For this review, use the dimensioned drawing (mm, ordinates from the lowest corner) and the shaded views. Give positions to 0.01 mm unless a question says otherwise; leave off trailing zeros. Order: outer loops, then holes, each group sorted by start corner. A loop starts at its lowest first (then second) coordinate and runs counter-clockwise, first axis right, second up. Notation, with made-up numbers: (10, 64) -> (68, 64) arc R19 ccw to (68, 98) -> close; hole circle Ø11 at (-32.5, -9). An arc over 180 degrees is marked (long way). Return JSON: item names as keys, results as strings.
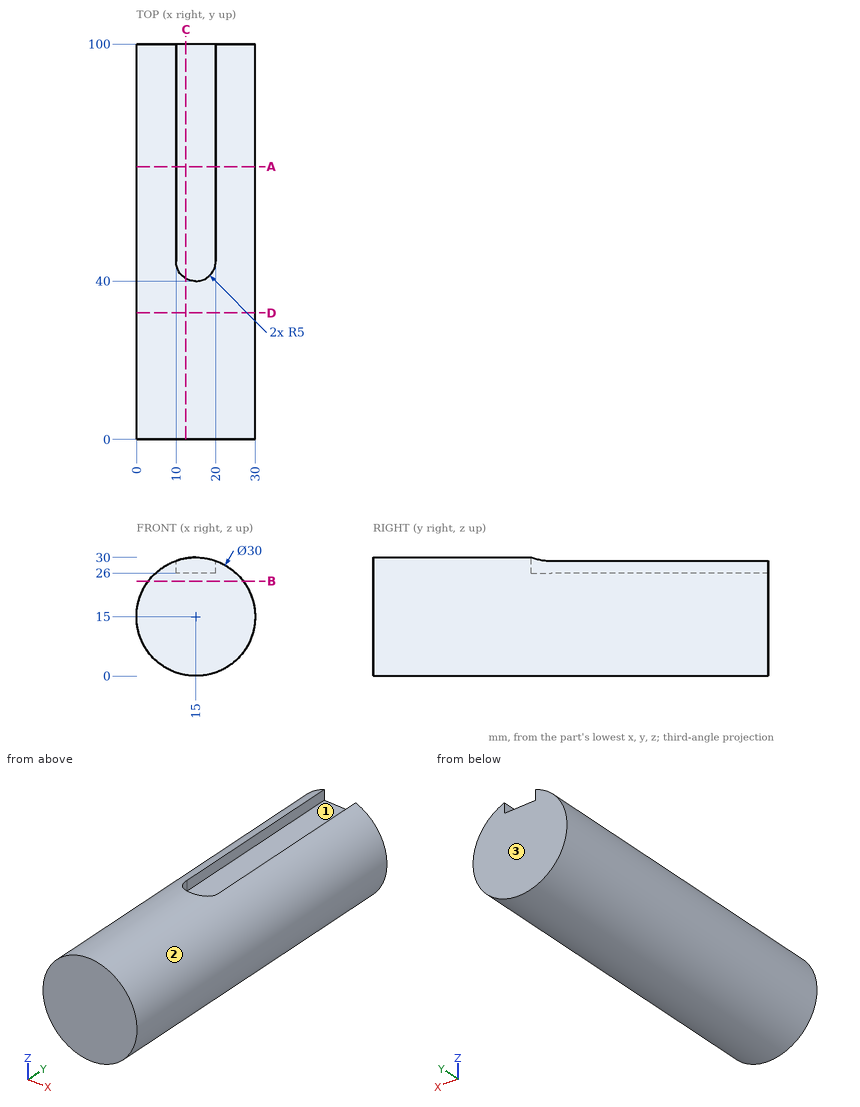
Item 1: Mouldability with a two-part tool opening along X and no side actions: class the marked faces 1, 2 and 3 as released by +X, released by -X, zero draft, split by the parting line, or undercut.
Result set:
{"face 1": "undercut", "face 2": "split by the parting line", "face 3": "zero draft"}
Item 2: Add section A-A (y = 69). Give the boundary of the cut face in (x, z), plus the area to 3 significant figures.
Result set:
{"outline": "(10, 26) -> (10, 29.14) arc R15 ccw (long way) to (20, 29.14) -> (20, 26) -> close", "area": "670 mm^2"}
Item 3: Add section D-D (y = 32). Give the boundary of the cut face in (x, z), plus the area to 3 significant figures.
Result set:
{"outline": "circle Ø30 at (15, 15)", "area": "707 mm^2"}
Item 4: Add section B-B (z = 24). Give the boundary of the cut face in (x, y).
Result set:
{"outline": "(3, 0) -> (27, 0) -> (27, 100) -> (3, 100) -> close"}
Item 5: Wall thickness on L1, parallel to Z at x = 14.5, y = 4; L2, parallel to X at y = 86.5, z = 4.5; L3, parallel to X at y = 37.5, z = 3: over which ranges is each line inside the solid? List them lowest first. Write a range as [from, to].
Result set:
{"L1": "z = [0.01, 29.99]", "L2": "x = [4.29, 25.71]", "L3": "x = [6, 24]"}
Item 6: Add section C-C (x = 12.5). Give the boundary of the cut face in (y, z), plus the area to 3 significant figures.
Result set:
{"outline": "(0, 0.21) -> (100, 0.21) -> (100, 26) -> (40.67, 26) -> (40.67, 29.79) -> (0, 29.79) -> close", "area": "2,730 mm^2"}
Item 7: For pin 1 (1 mm diameter, centred on y = 21, z = 8, fed in from -X); pin 2 (1.6 mm diameter, centred on y = 60, z = 27.5, fed in from -X); pin 3 (5 mm diameter, centred on y = 90, z = 5.5, fed in from -X); pin 4 (8 mm diameter, centred on x = 3.5, z = 3.5, fed in from +Y), all flat-tipped, find the tip position at first contact; note any pin that passes through.
Result set:
{"pin 1": "stops at x = 1.48", "pin 2": "stops at x = 5.61", "pin 3": "stops at x = 1.73", "pin 4": "stops at y = 100"}
